```python
from build123d import *

# Parameters (mm, degrees)
BOSS_EXTRUDE1_DEPTH     = 20
SKETCH2_R               = 2
CUT_EXTRUDE1_DEPTH      = 20
SKETCH3_W               = 2
SKETCH3_H               = 20
BOSS_EXTRUDE2_DEPTH     = 20
CUT_EXTRUDE2_DEPTH      = 60.712985217
CUT_EXTRUDE2_DEPTH_BACK = 60.712985217
SKETCH4_R               = 3


with BuildPart() as part:
    # Sketch1 → Boss-Extrude1 (new body)
    with BuildSketch(Plane.XY):
        Polygon((-8.296296296, 12.185185185), (-8.296296296, -32.814814815), (-6.296296296, -32.814814815), (-6.296296296, 10.185185185), (23.703703704, 10.185185185), (23.703703704, -7.814814815), (25.703703704, -7.814814815), (25.703703704, 12.185185185), align=None)
    extrude(amount=BOSS_EXTRUDE1_DEPTH)

    # Sketch2 → Cut-Extrude1 (cut)
    with BuildSketch(Plane(origin=(0, 12.185185185, 0), x_dir=(1, 0, 0), z_dir=(0, 1, 0))):
        with Locations(Location((13.703703704, -15, 0), (0, 0, 180))):
            Circle(SKETCH2_R)
        with Locations(Location((3.703703704, -5, 0), (0, 0, 180))):
            Circle(SKETCH2_R)
    extrude(amount=-CUT_EXTRUDE1_DEPTH, mode=Mode.SUBTRACT)

    # Sketch3 → Boss-Extrude2 (add)
    with BuildSketch(Plane(origin=(25.703703704, 0, 0), x_dir=(0, 0, -1), z_dir=(1, 0, 0))):
        with Locations((-19, 2.185185185)):
            Rectangle(SKETCH3_W, SKETCH3_H)
        with Locations((-1, 2.185185185)):
            Rectangle(SKETCH3_W, SKETCH3_H)
    extrude(amount=BOSS_EXTRUDE2_DEPTH)

    # Sketch4 → Cut-Extrude2 (cut, two sides: drawn at the far end of the back side and taken through both)
    with BuildSketch(Plane(origin=(0, 0, 0), x_dir=(-1, 0, 0), z_dir=(0, 0, -1)).offset(-CUT_EXTRUDE2_DEPTH_BACK)):
        with Locations((-35.703703704, 2.185185185)):
            Circle(SKETCH4_R)
    extrude(amount=CUT_EXTRUDE2_DEPTH + CUT_EXTRUDE2_DEPTH_BACK, mode=Mode.SUBTRACT)


solid = part.part
```
Can you work these out from the model? Positions are in its coordinate system, mm. A direction names the side the tool comes from. Give positions to 0.01 mm unless a question says otherwise; leave off trailing zeros. Write each loop counter-clockwise with the first axis right and the second up, starting at its lowest first coordinate (ties: lowest second). Pieces come first, ordered by that corner, then holes. Notation, with made-up numbers: (11, -1) -> (45, -1) arc R17 cw to (45, 19) -> close; hole circle Ø9 at (-9, -12.5). An arc over 180 degrees is marked (long way). Write item = value, one per line.
(1) I'm going to push flat-ended pins straight in: P1, Ø10, axis at y = -11.5, z = 7.5, coming from the +X side; P2, Ø10, axis at y = -28, z = 14.5, coming from the +X side. Where does each tip first touch, or does it pass through?
Worked out:
P1 = 25.7
P2 = -6.3
(2) I need wall thicknesses on probe 1 along Z at (x, y) = (35, -2.5); probe 2 along X at (y, z) = (-2, 10.25); probe 3 along Y at (x, z) = (-5, 18.75). Which ranges of each line are inside material? Lowest first, please. Write a range as from..to.
Worked out:
probe_1 = 0..2, 18..20
probe_2 = -8.3..-6.3, 23.7..25.7
probe_3 = 10.19..12.19
(3) Suppose I cut it at A-A on y = -5.5. Write out the boundary of the cut face in (x, z), then the cut area to 3 significant figures.
Worked out:
outline = (-8.3, 0) -> (-6.3, 0) -> (-6.3, 20) -> (-8.3, 20) -> close; (23.7, 0) -> (45.7, 0) -> (45.7, 2) -> (25.7, 2) -> (25.7, 18) -> (45.7, 18) -> (45.7, 20) -> (23.7, 20) -> close
area = 160 mm^2
(4) Suppose I cut it at C-C on z = 8. Write out the boundary of the cut face in (x, y), then the cut area to 3 significant figures.
Worked out:
outline = (-8.3, -32.81) -> (-6.3, -32.81) -> (-6.3, 10.19) -> (23.7, 10.19) -> (23.7, -7.81) -> (25.7, -7.81) -> (25.7, 12.19) -> (-8.3, 12.19) -> close
area = 190 mm^2
(5) Suppose I cut it at B-B on z = 15. Write out the boundary of the cut face in (x, y), then the cut area to 3 significant figures.
Worked out:
outline = (-8.3, -32.81) -> (-6.3, -32.81) -> (-6.3, 10.19) -> (11.7, 10.19) -> (11.7, 12.19) -> (-8.3, 12.19) -> close; (15.7, 10.19) -> (23.7, 10.19) -> (23.7, -7.81) -> (25.7, -7.81) -> (25.7, 12.19) -> (15.7, 12.19) -> close
area = 182 mm^2
(6) Thinking about a two-plate mould opening in X: for faces 4 (the face through (45.704, 2, 19)), 5 (the face through (13.964, 11.199, 16.983)), 6 (the face through (25, -7.815, 9)), which applies, released by +X, released by -X, zero draft, split by the parting line, or undercut?
Worked out:
face_4 = released by +X
face_5 = undercut
face_6 = zero draft
(7) Suppose I cut it at D-D on y = -16. Write out the boundary of the cut face in (x, z), then the cut area to 3 significant figures.
Worked out:
outline = (-8.3, 0) -> (-6.3, 0) -> (-6.3, 20) -> (-8.3, 20) -> close
area = 40.0 mm^2
(8) For faces 1 (the face through (33, 0, 2)), 2 (the face through (23.704, 1, 10)), 3 (the face through (12, 12.185, 10)), which set-ups out of +Z, -Z, +X, -X, +Y, -Y let a thin tool reach every point of the face, with its end or its side?
Worked out:
face_1 = +X, +Y, -Y
face_2 = +Z, -Z, -Y
face_3 = +Z, -Z, +X, -X, +Y
